from build123d import *

# Parameters (mm, degrees)
BOSS_EXTRUDE1_DEPTH = 320
SKETCH2_W           = 390.491901408
SKETCH2_H           = 141.475704226
BOSS_EXTRUDE2_DEPTH = 20
SKETCH4_W           = 300
SKETCH4_H           = 300
CUT_EXTRUDE1_DEPTH  = 100
SKETCH5_W           = 20
SKETCH5_H           = 20
BOSS_EXTRUDE3_DEPTH = 5
SKETCH6_W           = 15
SKETCH6_H           = 15
BOSS_EXTRUDE4_DEPTH = 5
SKETCH7_W           = 10
SKETCH7_H           = 10
BOSS_EXTRUDE6_DEPTH = 20
BOSS_EXTRUDE7_REACH = 252.246
SKETCH8_W           = 10
SKETCH8_H           = 10


with BuildPart() as part:
    # Sketch1 → Boss-Extrude1 (new body)
    with BuildSketch(Plane.XY):
        Polygon((-180.245950704, 55.737852113), (179.754049296, 55.737852113), (179.754049296, 15.737852113), (159.754049296, 15.737852113), (159.754049296, -14.262147887), (179.754049296, -14.262147887), (179.754049296, -54.262147887), (-180.245950704, -54.262147887), (-180.245950704, -14.262147887), (-160.245950704, -14.262147887), (-160.245950704, 15.737852113), (-180.245950704, 15.737852113), align=None)
    extrude(amount=-BOSS_EXTRUDE1_DEPTH)

    # Sketch2 → Boss-Extrude2 (add)
    with BuildSketch(Plane.XY):
        Rectangle(SKETCH2_W, SKETCH2_H)
    extrude(amount=BOSS_EXTRUDE2_DEPTH)

    # Sketch4 → Cut-Extrude1 (cut)
    with BuildSketch(Plane(origin=(0, 55.737852113, 0), x_dir=(1, 0, 0), z_dir=(0, 1, 0))):
        with Locations((-0.245950704, 150)):
            Rectangle(SKETCH4_W, SKETCH4_H)
    extrude(amount=-CUT_EXTRUDE1_DEPTH, mode=Mode.SUBTRACT)

    # Sketch5 → Boss-Extrude3 (add)
    with BuildSketch(Plane.XY.offset(20)):
        with Locations((-60, 2.912454094)):
            Rectangle(SKETCH5_W, SKETCH5_H)
        with Locations((60, 2.912454094)):
            Rectangle(SKETCH5_W, SKETCH5_H)
    extrude(amount=BOSS_EXTRUDE3_DEPTH)

    # Sketch6 → Boss-Extrude4 (add)
    with BuildSketch(Plane.XY.offset(25)):
        with Locations((-60, 2.912454094)):
            Rectangle(SKETCH6_W, SKETCH6_H)
        with Locations((60, 2.912454094)):
            Rectangle(SKETCH6_W, SKETCH6_H)
    extrude(amount=BOSS_EXTRUDE4_DEPTH)

    # Sketch7 → Boss-Extrude6 (add)
    with BuildSketch(Plane.XY.offset(30)):
        with Locations((-60, 2.912454094)):
            Rectangle(SKETCH7_W, SKETCH7_H)
        with Locations((60, 2.912454094)):
            Rectangle(SKETCH7_W, SKETCH7_H)
    extrude(amount=BOSS_EXTRUDE6_DEPTH)

    # Sketch8 → Boss-Extrude7 (add, up to next)
    with BuildSketch(Plane.ZY.offset(-55), mode=Mode.PRIVATE) as boss_extrude7_sk1:
        with Locations((45, 2.912454094)):
            Rectangle(SKETCH8_W, SKETCH8_H)
    boss_extrude7_tool1 = extrude(boss_extrude7_sk1.sketch, amount=BOSS_EXTRUDE7_REACH, mode=Mode.PRIVATE) - part.part
    add(boss_extrude7_tool1.solids().sort_by_distance((55, 2.912454, 45))[0])


solid = part.part
Source: CAD feature listing. Evaluate the final solid. Frame: model axes, mm. A direction names the side the tool comes from. Give positions to 0.01 mm unless a question says otherwise; leave off trailing zeros. Write each loop counter-clockwise with the first axis right and the second up, starting at its lowest first coordinate (ties: lowest second). Pieces come first, ordered by that corner, then holes. Notation, with made-up numbers: M -0.5,-20 L 25.5,-20 A26 cw 25.5,7 Z; hole C 52,21.25 d7. An arc over 180 degrees is marked long. Return JSON: item names as keys, results as strings. Group by question number.
1) Material intervals for line 1 along Z through (x, y) = (72.5, -28); line 2 along X through (y, z) = (-18.5, -169.5); line 3 along Y through (x, z) = (-175, -226), sorted ascending. Write a range as [from, to].
2) Cut plane D-D, the plane x = 121.5. Output: boundary loops of the cut face in (y, z), plus the area to 3 significant figures.
3) Pin query (flat end, axial travel): P1, Ø22, axis at x = -173, z = -182, coming from the +Y side; P2, Ø10, axis at y = 37.5, z = -178.5, coming from the +X side; P3, Ø1.5, axis at x = 57.5, z = 28, coming from the -Y side. Return the tip coordinate at first contact, or that it passes through.
4) Cut plane C-C, the plane z = -55. Output: boundary loops of the cut face in (x, y).
5) Pull-direction query (Z, two-part tool) for faces 1 (the face through (-3, 70.738, 10)), 2 (the face through (1, 3, 50)), 3 (the face through (149.754, 6, -148)), 4 (the face through (1, 3, 40)); classes: pulls with the +Z half, pulls with the -Z half, needs draft (parallel to the pull), parting line crosses it, or undercut.
6) Cut plane A-A, the plane x = 22. Output: boundary loops of the cut face in (y, z), plus the area to 3 significant figures.
7) Cut plane B-B, the plane y = -32.5. Output: boundary loops of the cut face in (x, z), plus the area to 3 significant figures.
8) Set-up query: faces 5 (the face through (1, -2.088, 44)), 6 (the face through (-170, -14.262, -158)), 7 (the face through (2, -54.262, -158)), 8 (the face through (-180.246, 35, -158)), 9 (the face through (1, 7.912, 44)). Return all of +Z, -Z, +X, -X, +Y, -Y with unobstructed straight access to the full face (end or side cutting, diameter ignored); none if empty.
Recorded:
{
 "1": {"line 1": "z = [-320, -300], [0, 20]", "line 2": "x = [-180.25, -150.25], [149.75, 179.75]", "line 3": "y = [-54.26, -14.26], [15.74, 55.74]"},
 "2": {"outline": "M -70.74,0 L -54.26,0 L -54.26,-320 L 55.74,-320 L 55.74,-300 L -44.26,-300 L -44.26,0 L 70.74,0 L 70.74,20 L -70.74,20 Z", "area": "8,030 mm²"},
 "3": {"P1": "stops at y = 55.74", "P2": "stops at x = 179.75", "P3": "stops at y = -4.59"},
 "4": {"outline": "M -180.25,-54.26 L 179.75,-54.26 L 179.75,-14.26 L 159.75,-14.26 L 159.75,15.74 L 179.75,15.74 L 179.75,55.74 L 149.75,55.74 L 149.75,-44.26 L -150.25,-44.26 L -150.25,55.74 L -180.25,55.74 L -180.25,15.74 L -160.25,15.74 L -160.25,-14.26 L -180.25,-14.26 Z"},
 "5": {"face 1": "needs draft", "face 2": "pulls with the +Z half", "face 3": "undercut", "face 4": "undercut"},
 "6": {"outline": "M -70.74,0 L -54.26,0 L -54.26,-320 L 55.74,-320 L 55.74,-300 L -44.26,-300 L -44.26,0 L 70.74,0 L 70.74,20 L -70.74,20 Z; M -2.09,40 L 7.91,40 L 7.91,50 L -2.09,50 Z", "area": "8,130 mm²"},
 "7": {"outline": "M -195.25,0 L -180.25,0 L -180.25,-320 L 179.75,-320 L 179.75,0 L 195.25,0 L 195.25,20 L -195.25,20 Z; hole M -150.25,-300 L 149.75,-300 L 149.75,0 L -150.25,0 Z", "area": "33,000 mm²"},
 "8": {"face 5": "+Z, +X, -X, -Y", "face 6": "-Z, -X", "face 7": "-Z, +X, -X, -Y", "face 8": "-Z, -X, +Y, -Y", "face 9": "+Z, +X, -X, +Y"}
}
